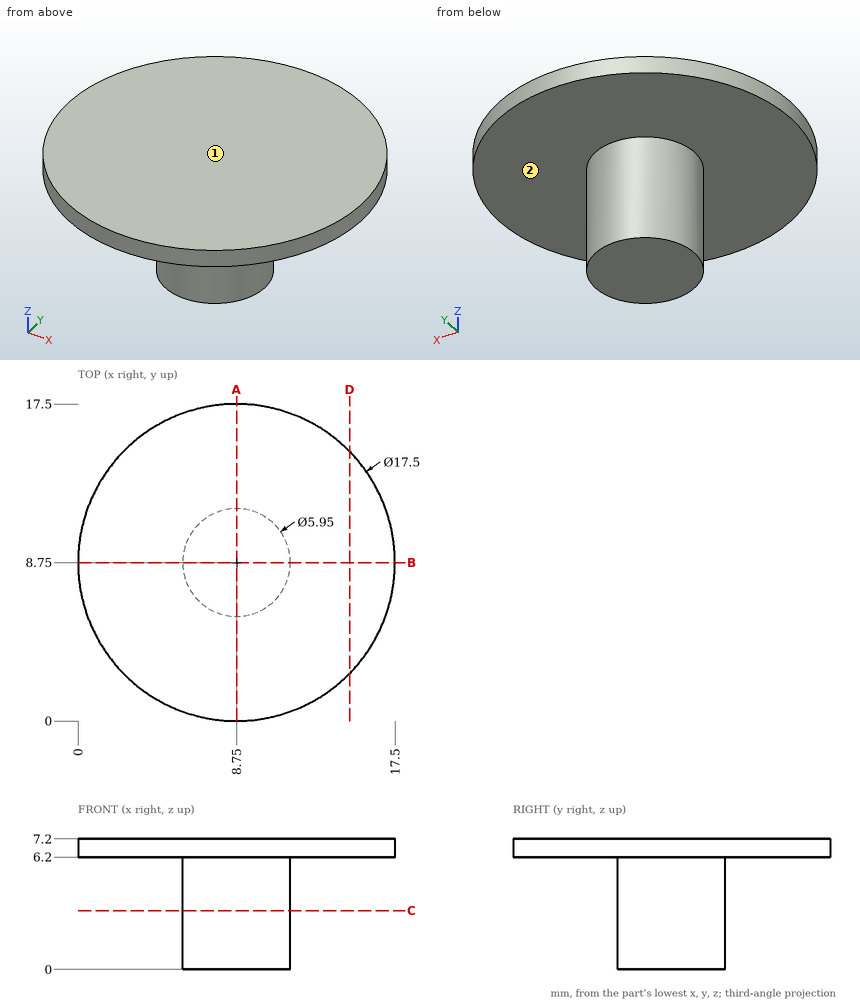
Print and shaded views of the part. All mm, measured from the part's lowest x, y and z. A direction names the side the tool comes from. Give positions to 0.01 mm unless a question says otherwise; leave off trailing zeros. Write each loop counter-clockwise with the first axis right and the second up, starting at its lowest first coordinate (ties: lowest second). Pieces come first, ordered by that corner, then holes. Notation, with made-up numbers: (-13.75, 6) -> (43.25, 6) arc R19 ccw to (43.25, 16) -> close; hole circle Ø4 at (-31.5, 71.25). An arc over 180 degrees is marked (long way). Write each question's results on one line, items separated by ' | '.
1. Cut at A-A, the plane x = 8.75. Write the cut outline in (y, z) (3 decimals).
Geometry check:
outline: (0, 6.2) -> (5.775, 6.2) -> (5.775, 0) -> (11.725, 0) -> (11.725, 6.2) -> (17.5, 6.2) -> (17.5, 7.2) -> (0, 7.2) -> close
2. Which spindle directions (+Z, -Z, +X, -X, +Y, -Y) get a long thin tool onto all of the face, cutting with end or side? Do the marked faces 1 and 2. Say none if no direction does.
Geometry check:
face 1: +Z, +X, -X, +Y, -Y | face 2: -Z
3. Drop flat-ended pins along their axis: P1, Ø1, axis at x = 3.5, z = 5, coming from the -Y side; P2, Ø2, axis at y = 10.5, z = 3.5, coming from the +X side. Give the stop position or say it passes through.
Geometry check:
P1: through | P2: x = 11.63
4. Cut at C-C, the plane z = 3.25. Write the cut outline in (x, y) (3 decimals).
Geometry check:
outline: circle Ø5.95 at (8.75, 8.75)
5. Wall check: probe 1 along Z at (x, y) = (5, 12.75); probe 2 along Y at (x, z) = (10.75, 6.25); probe 3 along X at (y, z) = (10, 3.75). Give the ranges that are in metal, low to high. Write a range as [from, to].
Geometry check:
probe 1: [6.2, 7.2] | probe 2: [0.23, 17.27] | probe 3: [6.05, 11.45]
6. Cut at D-D, the plane x = 15. Write the cut outline in (y, z), then the cut area to 3 significant figures.
Geometry check:
outline: (2.63, 6.2) -> (14.87, 6.2) -> (14.87, 7.2) -> (2.63, 7.2) -> close | area: 12.2 mm²
